from build123d import *

# Parameters (mm, degrees)
SKETCH_1_W          = 28.6
SKETCH_1_H          = 30
EXTRUDE_1_DEPTH     = 3
SKETCH_1_4_W        = 28.6
SKETCH_1_4_H        = 30
SKETCH_1_4_W_2      = 25
SKETCH_1_4_H_2      = 24
EXTRUDE_2_DEPTH     = 8
SKETCH_2_W          = 22
SKETCH_2_H          = 3
CUT_EXTRUDE_1_DEPTH = 8
SKETCH_3_W          = 25
SKETCH_3_H          = 6
CUT_EXTRUDE_2_DEPTH = 2
SKETCH_4_R          = 0.9
EXTRUDE_3_DEPTH     = 2


with BuildPart() as part:
    # Sketch 1 → Extrude 1 (new body)
    with BuildSketch(Plane(origin=(0, 0, 0), x_dir=(1, 0, 0), z_dir=(0, 1, 0))):
        Rectangle(SKETCH_1_W, SKETCH_1_H)
    extrude(amount=EXTRUDE_1_DEPTH)

    # Sketch 1_4 → Extrude 2 (add)
    with BuildSketch(Plane(origin=(0, 0, 0), x_dir=(1, 0, 0), z_dir=(0, 1, 0))):
        Rectangle(SKETCH_1_4_W, SKETCH_1_4_H)
        Rectangle(SKETCH_1_4_W_2, SKETCH_1_4_H_2, mode=Mode.SUBTRACT)
    extrude(amount=EXTRUDE_2_DEPTH)

    # Sketch 2 → Cut-Extrude 1 (cut)
    with BuildSketch(Plane(origin=(0, 8, 0), x_dir=(1, 0, 0), z_dir=(0, 1, 0))):
        with Locations((0, -13.5)):
            Rectangle(SKETCH_2_W, SKETCH_2_H)
    extrude(amount=-CUT_EXTRUDE_1_DEPTH, mode=Mode.SUBTRACT)

    # Sketch 3 → Cut-Extrude 2 (cut)
    with BuildSketch(Plane(origin=(0, 3, 0), x_dir=(1, 0, 0), z_dir=(0, 1, 0))):
        with Locations((0, -9)):
            Rectangle(SKETCH_3_W, SKETCH_3_H)
    extrude(amount=-CUT_EXTRUDE_2_DEPTH, mode=Mode.SUBTRACT)

    # Sketch 4 → Extrude 3 (add)
    with BuildSketch(Plane(origin=(0, 3, 0), x_dir=(1, 0, 0), z_dir=(0, 1, 0))):
        with Locations(Location((-10.5, 9.8, 0), (0, 0, 90))):
            Circle(SKETCH_4_R)
        with Locations(Location((-10.5, -2.6, 0), (0, 0, 90))):
            Circle(SKETCH_4_R)
        with Locations(Location((10.5, 9.8, 0), (0, 0, 90))):
            Circle(SKETCH_4_R)
        with Locations(Location((10.5, -2.6, 0), (0, 0, 90))):
            Circle(SKETCH_4_R)
    extrude(amount=EXTRUDE_3_DEPTH)


solid = part.part
The listing builds one solid part. Answer for the finished solid, in the listing's coordinates (mm). A direction names the side the tool comes from. Give positions to 0.01 mm unless a question says otherwise; leave off trailing zeros. Order: outer loops, then holes, each group sorted by start corner. A loop starts at its lowest first (then second) coordinate and runs counter-clockwise, first axis right, second up. Notation, with made-up numbers: (57, 53.5) -> (83, 53.5) arc R12 cw to (83, 63.5) -> close; hole circle Ø10 at (30.5, 23.25). An arc over 180 degrees is marked (long way). Put each result on its own line as item: value.
Item 1: For a pull along Z with two mould halves and no side action, classify faces 3 (the face through (0, 3, -3)), 4 (the face through (-11, 4, 14)), 5 (the face through (-13, 4, 15)) as released by +Z, released by -Z, zero draft, split by the parting line, or undercut.
Established:
face 3: undercut
face 4: zero draft
face 5: released by +Z
Item 2: A cutting plane is placed at B-B on x = -10.5. Give the vertices of the cut face in (y, z).
Established:
outline: (0, -15) -> (8, -15) -> (8, -12) -> (3, -12) -> (3, -10.7) -> (5, -10.7) -> (5, -8.9) -> (3, -8.9) -> (3, 1.7) -> (5, 1.7) -> (5, 3.5) -> (3, 3.5) -> (3, 6) -> (1, 6) -> (1, 12) -> (0, 12) -> close
Item 3: Given P1, Ø1, axis at x = -3.5, y = 2.5, coming from the +Z side; P2, Ø2, axis at x = -10.5, z = 2.5, coming from the +Y side; P3, Ø1.5, axis at x = 4, y = 1, coming from the +Z side, each flat-ended and moving along its own axis, determine where each tip first touches the part or whether it passes through.
Established:
P1: stops at z = 6
P2: stops at y = 5
P3: stops at z = 12
Item 4: A cutting plane is placed at A-A on y = 3.5. Give the vertices of the cut face in (x, z), plus the area to 3 significant figures.
Established:
outline: (-14.3, -15) -> (14.3, -15) -> (14.3, 15) -> (11, 15) -> (11, 12) -> (12.5, 12) -> (12.5, -12) -> (-12.5, -12) -> (-12.5, 12) -> (-11, 12) -> (-11, 15) -> (-14.3, 15) -> close; circle Ø1.8 at (-10.5, -9.8); circle Ø1.8 at (-10.5, 2.6); circle Ø1.8 at (10.5, -9.8); circle Ø1.8 at (10.5, 2.6)
area: 202 mm^2
Item 5: For faces 1 (the face through (-14.3, 4, 0)), 2 (the face through (0, 5, -12)), determine the directions among +Z, -Z, +X, -X, +Y, -Y from which every point of the face is accessible in a straight line to the end or side of a thin tool.
Established:
face 1: +Z, -Z, -X, +Y, -Y
face 2: +Y
Item 6: Straight lines are drawn through the part: line 1 (X direction, y = 6.5, z = -9.5); line 2 (X direction, y = 4.25, z = 13.25); line 3 (Z direction, x = 4.5, y = 6.5). For each, find the intervals that lie inside material, in ascending order.
Established:
line 1: x = -14.3 to -12.5, 12.5 to 14.3
line 2: x = -14.3 to -11, 11 to 14.3
line 3: z = -15 to -12
Item 7: A cutting plane is placed at D-D on z = 2.6. Give the vertices of the cut face in (x, y).
Established:
outline: (-14.3, 0) -> (14.3, 0) -> (14.3, 8) -> (12.5, 8) -> (12.5, 3) -> (11.4, 3) -> (11.4, 5) -> (9.6, 5) -> (9.6, 3) -> (-9.6, 3) -> (-9.6, 5) -> (-11.4, 5) -> (-11.4, 3) -> (-12.5, 3) -> (-12.5, 8) -> (-14.3, 8) -> close
Item 8: A cutting plane is placed at C-C on z = 12.75. Give the vertices of the cut face in (x, y).
Established:
outline: (-14.3, 0) -> (-11, 0) -> (-11, 8) -> (-14.3, 8) -> close; (11, 0) -> (14.3, 0) -> (14.3, 8) -> (11, 8) -> close
